```python
from build123d import *

# Parameters (mm, degrees)
F1_DEPTH = 25.4
F2_R     = 5.08
F3_T     = -2.54


with BuildPart() as f1:
    # F0 (on Top) → F1 (new body)
    with BuildSketch(Plane.XY):
        Polygon((-13.158648, 54.746445), (-35.605059, 27.995854), (-20.167736, -59.553555), (30.632264, -59.553555), (46.069587, 27.995854), (23.623176, 54.746445), align=None)
    extrude(amount=F1_DEPTH)

    # F2
    f2_edges = [f1.edges().sort_by_distance(p)[0] for p in [
        (-27.886397, -15.77885, 0),
        (5.232264, -59.553555, 0),
        (38.350926, -15.77885, 0),
        (34.846382, 41.37115, 0),
        (5.232264, 54.746445, 0),
        (-24.381853, 41.37115, 0),
    ]]
    fillet(f2_edges, radius=F2_R)

    # F3
    f3_openings = [f1.faces().sort_by_distance(p)[0] for p in [
        (5.232264, -1.206794, 25.4),
    ]]
    offset(amount=F3_T, openings=f3_openings)


solid = f1.part
```
Could you check a few things on this model? Use its own coordinates, in mm. A direction names the side the tool comes from. Coordinates: 2 decimals unless noted, no trailing zeros. Loops run counter-clockwise (first coordinate to the right, second up) from the corner with the lowest first, then second, coordinate; pieces in that order, holes last.
1) Imagine slicing it at B-B (x = 18.5). List the corners of the cut face in (y, z) for me.
Reported:
outline: (-59.55, 5.08) arc R5.08 ccw to (-54.47, 0) - (49.67, 0) arc R5.08 ccw to (54.75, 5.08) - (54.75, 25.4) - (52.21, 25.4) - (52.21, 5.08) arc R2.54 cw to (49.67, 2.54) - (-54.47, 2.54) arc R2.54 cw to (-57.01, 5.08) - (-57.01, 25.4) - (-59.55, 25.4) - close
2) Thinking about a two-plate mould opening in X: for faces 1 (the face through (35.004, 41.184, 15.098)), 2 (the face through (32.199, 39.447, 3.304)), 3 (the face through (5.588, -58.105, 1.528)), which applies, released by +X, released by -X, zero draft, split by the parting line, or undercut?
Reported:
face 1: released by +X
face 2: undercut
face 3: zero draft
3) Imagine slicing it at A-A (z = 7.5). List the corners of the cut face in (x, y) for me.
Reported:
outline: (-35.61, 28) - (-20.17, -59.55) - (30.63, -59.55) - (46.07, 28) - (23.62, 54.75) - (-13.16, 54.75) - close; hole (-32.9, 27.27) - (-18.04, -57.01) - (28.5, -57.01) - (43.36, 27.27) - (22.44, 52.21) - (-11.97, 52.21) - close
4) Please list where these lines run through material, in increasing order: line 1 along Y through (x, z) = (14.5, 7); line 2 along Z through (x, y) = (31, -17.5); line 3 along X through (y, z) = (14, 9.75).
Reported:
line 1: y = -59.55 to -57.01, 52.21 to 54.75
line 2: z = 0 to 2.54
line 3: x = -33.14 to -30.56, 41.02 to 43.6
5) Which directions (+Z, -Z, +X, -X, +Y, -Y) give clear straight access to the entire face, cutting with the end or side of a thin tool? Please do faces 4 (the face through (37.032, -14.914, 1.528)), 5 (the face through (5.558, -56.289, 3.304)).
Reported:
face 4: -Z, +X, -Y
face 5: +Z
6) Will these pins go through, and if not, where does the flat tip stop? pin 1 Ø6 at (y, z) = (-6.5, 15) entering from -X; pin 2 Ø3 at (y, z) = (-13, 17) entering from -X; pin 3 Ø10 at (y, z) = (-39.5, 10) entering from +X.
Reported:
pin 1: stops at x = -30.05
pin 2: stops at x = -28.64
pin 3: stops at x = 35.05
